from build123d import *

# Parameters (mm, degrees)
F0_R     = 10.7945636434
F0_R_2   = 9.5
F1_DEPTH = 4
F2_W     = 2.2937387829
F2_H     = 8.5183947237
F3_DEPTH = 4
F4_R     = 0.6


with BuildPart() as f1:
    # F0 (on Top) → F1 (new body)
    with BuildSketch(Plane.XY):
        with Locations((-12.9060586914, -22.1966579556)):
            Circle(F0_R)
        with Locations((-12.9060586914, -22.1966579556)):
            Circle(F0_R_2, mode=Mode.SUBTRACT)
    extrude(amount=F1_DEPTH)

    # F2 (on face) → F3 (join)
    with BuildSketch(Plane.XY.offset(4)):
        with Locations((-23.9716902075, -22.1966579556)):
            Rectangle(F2_W, F2_H)
        Polygon((-25.1185595989, -17.9374605938), (-22.824820816, -17.9374605938), (-18.1995894648, -12.7891537062), align=None)
        Polygon((-18.1995894648, -31.6041622051), (-22.824820816, -26.4558553175), (-25.1185595989, -26.4558553175), align=None)
    extrude(amount=-F3_DEPTH)

    # F4
    f4_edges = [f1.edges().sort_by_distance(p)[0] for p in [
        (-2.111495, -22.196658, 4),
        (-2.111495, -22.196658, 0),
        (-22.75742, -28.212746, 0),
        (-25.11856, -22.196658, 4),
        (-22.75742, -16.18057, 4),
        (-25.11856, -22.196658, 0),
        (-22.75742, -16.18057, 0),
        (-22.406059, -22.196658, 4),
        (-22.406059, -22.196658, 0),
        (-25.11856, -26.455855, 2),
        (-25.11856, -17.937461, 2),
        (-20.39628, -14.42368, 2),
        (-20.39628, -29.969636, 2),
        (-22.75742, -28.212746, 4),
    ]]
    fillet(f4_edges, radius=F4_R)


solid = f1.part
Work out the finished part from the listing and answer in its coordinate system (mm). Give positions to 0.01 mm unless a question says otherwise; leave off trailing zeros. Write each loop counter-clockwise with the first axis right and the second up, starting at its lowest first coordinate (ties: lowest second). Pieces come first, ordered by that corner, then holes. Notation, with made-up numbers: M -37.5,79.5 L 0.5,79.5 A20 ccw 0.5,83.5 Z; hole C 1.5,21 d1. An arc over 180 degrees is marked long. Answer as CSV lines item,"result".
Q1. Find the intervals of material crossed by probe 1 along Y at (x, z) = (-13, 3.4); probe 2 along Y at (x, z) = (-11, 2.55); probe 3 along X at (y, z) = (-25, 3.8), in increasing order. Write a range as [from, to].
A:
probe 1,"y = [-32.99, -31.7], [-12.7, -11.4]"
probe 2,"y = [-32.82, -31.5], [-12.89, -11.57]"
probe 3,"x = [-24.97, -22.14], [-3.67, -2.64]"
Q2. A cutting plane is placed at A-A on z = 2.95. Write down the section's boundary in (x, y), plus the area to 3 significant figures.
A:
outline,"M -25.12,-26.15 A0.6 ccw -24.88,-26.64 L -20.43,-29.95 A0.6 cw -20.37,-30 A10.79 ccw long -20.37,-14.4 A0.6 cw -20.43,-14.45 L -24.88,-17.76 A0.6 ccw -25.12,-18.24 Z; hole C -12.91,-22.2 d19"
area,"104 mm²"
Q3. The mould has two halves that part along X. Classify faces 1 (the cylindrical face through (-22.575, -16.27, 0.171)), 2 (the cylindrical face through (-8.522, -30.625, 1.98)), 3 (the flat face through (-23.4, -21.4, 0)): +X half, -X half, draft (parallel to the pull), parting line (faces both ways), or undercut.
A:
face 1,"-X half"
face 2,"undercut"
face 3,"draft"
Q4. Given P1, Ø4, axis at x = -5, y = -23, coming from the -Z side; P2, Ø6, axis at x = -6.5, y = -13.5, coming from the +Z side, each flat-ended and moving along its own axis, determine where each tip first touches the part or whether it passes through.
A:
P1,"stops at z = 0.02"
P2,"stops at z = 4"
